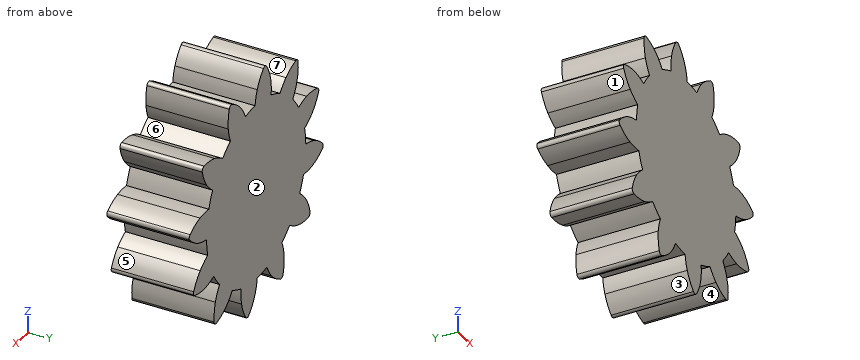
```python
from build123d import *

# Parameters (mm, degrees)
F1_DEPTH = 25
F2_COUNT = 12


with BuildPart() as f1:
    # F0 (on Front) → F1 (new body)
    with BuildSketch(Plane.XZ):
        with BuildLine():
            ThreePointArc((-7.9477143302, 30.5472248468), (-8.2259408607, 28.1405650395), (-8.1327613443, 25.7196687162))
            ThreePointArc((-8.1327613443, 25.7196687162), (-3.8188440215, 26.7031757717), (0.5978189292, 26.9682364733))
            ThreePointArc((0.5978189292, 26.9682364733), (0.1710931502, 29.1900709912), (-0.5687537498, 31.3281238622))
            ThreePointArc((-0.5687537498, 31.3281238622), (-2.0216895742, 33.8802868431), (-3.9594054698, 36.087052689))
            ThreePointArc((-3.9594054698, 36.087052689), (-4.8361287947, 36.3983837804), (-5.6282667199, 35.9104408081))
            ThreePointArc((-5.6282667199, 35.9104408081), (-7.0611591635, 33.3469709651), (-7.9477143302, 30.5472248468))
        make_face()
        with BuildLine():
            ThreePointArc((0.5978189292, 26.9682364733), (-3.8188440215, 26.7031757717), (-8.1327613443, 25.7196687162))
            ThreePointArc((-8.1327613443, 25.7196687162), (-15.9415032716, -21.760322594), (26.9748617412, 0))
            ThreePointArc((26.9748617412, 0), (19.2843103184, 18.8615625412), (0.5978189292, 26.9682364733))
        make_face()
    extrude(amount=F1_DEPTH)

    # F2: F1 ×12 about axis
    f2_axis = Axis((0, 0, 0), (0, 1, 0))


with BuildPart() as f1_1:
    add(f1.part)
    for i in range(1, F2_COUNT):
        add(f1.part.rotate(f2_axis, i * 360 / F2_COUNT))


solid = f1_1.part
```
Geometry check sheet. Reference: the model listing, model coordinates, mm. Face numbers are marked on the shaded views. A direction names the side the tool comes from. Coordinates: 2 decimals unless noted, no trailing zeros. Order: outer loops, then holes, each group sorted by start corner. A loop starts at its lowest first (then second) coordinate and runs counter-clockwise, first axis right, second up. Notation, with made-up numbers: M -31.5,-11.75 L -9.5,-11.75 A12 ccw -9.5,3.25 Z; hole C 20.25,57.25 d4. An arc over 180 degrees is marked long. One line per question, with ' | ' between items. Start each with the question number.
Item 1: Cross-section at A-A on z = 9.5. Enter the section's corners in (x, y).
Item 2: Cross-section at B-B on x = 3. Enter the section's corners in (y, z), then the cut area to 3 significant figures.
Item 3: Draft check along Z on the marked faces 1, 2 and 3. Enter one of: pulls with the +Z half, pulls with the -Z half, needs draft (parallel to the pull), parting line crosses it, or undercut.
Item 4: Material ranges on L1, parallel to Z at x = -27.5, y = -7; L2, parallel to Z at x = -31, y = -19.25; L3, parallel to X at y = -20.5, z = 31.5, recorded low to high. Write a range as [from, to].
Item 5: Gauge pin test, flat ends, axial feed: pin 1 (6 mm diameter, centred on x = -19, y = -9, fed in from +Z); pin 2 (5 mm diameter, centred on x = -4.5, z = 12, fed in from +Y); pin 3 (5 mm diameter, centred on y = -22.5, z = -15, fed in from -X); pin 4 (6 mm diameter, centred on x = -15, y = -5, fed in from +Z). Record the tip position at first contact, or that the pin passes through.
Item 6: Set-up check for the marked faces 4, 5, 6 and 7: record each of +Z, -Z, +X, -X, +Y, -Y from which the full face is reachable in a straight line by a thin tool's end or side.
Findings:
1) outline: M -31.54,-25 L 25.25,-25 L 25.25,0 L -31.54,0 Z
2) outline: M -25,-35.11 L 0,-35.11 L 0,26.81 L -25,26.81 Z | area: 1,550 mm²
3) face 1: undercut | face 2: needs draft | face 3: pulls with the -Z half
4) L1: z = [-22.88, -17.13], [-8.24, 0.53], [6.38, 15.18] | L2: z = [-7.85, -0.43], [8.93, 15.11] | L3: x = [-7.72, -0.65], [9.45, 15.03]
5) pin 1: stops at z = 29.31 | pin 2: stops at y = 0 | pin 3: stops at x = -27.72 | pin 4: stops at z = 27.99
6) face 4: -Z, +Y, -Y | face 5: +X, +Y, -Y | face 6: +Y, -Y | face 7: +Z, +Y, -Y
